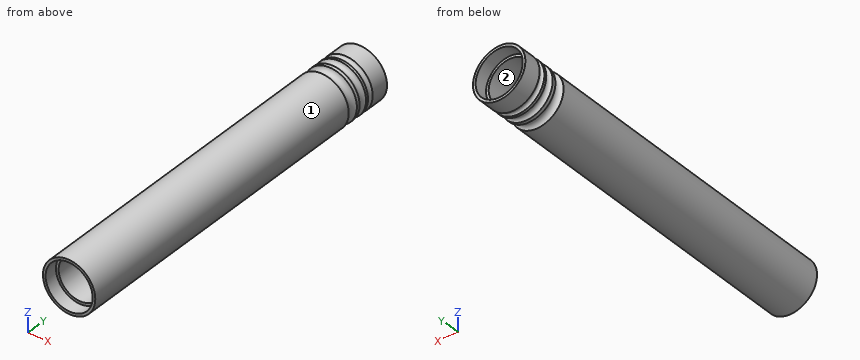
```python
from build123d import *

# Parameters (mm, degrees)
F0_R     = 25
F0_R_2   = 20
F1_DEPTH = 350
F2_R     = 22.5
F2_R_2   = 20
F3_DEPTH = 12.5
F4_R     = 22.5
F4_R_2   = 20
F5_DEPTH = 12.5
F6_R     = 3
F6_R_2   = 4
F6_R_3   = 5


with BuildPart() as f1:
    # F0 (on Front) → F1 (new body)
    with BuildSketch(Plane.XZ):
        Circle(F0_R)
        Circle(F0_R_2, mode=Mode.SUBTRACT)
    extrude(amount=F1_DEPTH)

    # F2 (on face) → F3 (cut)
    with BuildSketch(Plane.XZ.offset(350)):
        Circle(F2_R)
        Circle(F2_R_2, mode=Mode.SUBTRACT)
    extrude(amount=-F3_DEPTH, mode=Mode.SUBTRACT)

    # F4 (on face) → F5 (cut)
    with BuildSketch(Plane(origin=(0, 0, 0), x_dir=(-1, 0, 0), z_dir=(0, 1, 0))):
        Circle(F4_R)
        Circle(F4_R_2, mode=Mode.SUBTRACT)
    extrude(amount=-F5_DEPTH, mode=Mode.SUBTRACT)

    # F6 (on Right) → F7 (revolve, cut)
    with BuildSketch(Plane.YZ):
        with Locations((-20, 26)):
            Circle(F6_R)
        with Locations((-29, 26)):
            Circle(F6_R_2)
        with Locations((-41, 26)):
            Circle(F6_R_3)
    revolve(axis=Axis((0, 0, 0), (0, 1, 0)), mode=Mode.SUBTRACT)


solid = f1.part
```
Geometry check sheet. Reference: the model listing, model coordinates, mm. Face numbers are marked on the shaded views. Round coordinates to 2 decimals unless told otherwise and drop trailing zeros. Loops run counter-clockwise (first coordinate to the right, second up) from the corner with the lowest first, then second, coordinate; pieces in that order, holes last. Notation, with made-up numbers: (84, 57) - (111, 57) arc R22 cw to (111, 88) - close; hole circle Ø6 at (42, 55). An arc over 180 degrees is marked (long way). Use a Markdown table: item, result.
Q1. Cross-section at C-C on y = -153. Record the cut outline in (x, z), plus the area to 3 significant figures.
Solutions:
| item | result |
|---|---|
| outline | circle Ø50 at (0, 0); hole circle Ø40 at (0, 0) |
| area | 707 mm2 |
Q2. Cross-section at A-A on x = 0. Record the cut outline in (y, z).
Solutions:
| item | result |
|---|---|
| outline | (-350, -25) - (-45.9, -25) arc R5 cw to (-36.1, -25) - (-32.87, -25) arc R4 cw to (-25.13, -25) - (-22.83, -25) arc R3 cw to (-17.17, -25) - (0, -25) - (0, -22.5) - (-12.5, -22.5) - (-12.5, -20) - (-337.5, -20) - (-337.5, -22.5) - (-350, -22.5) - close; (-350, 22.5) - (-337.5, 22.5) - (-337.5, 20) - (-12.5, 20) - (-12.5, 22.5) - (0, 22.5) - (0, 25) - (-17.17, 25) arc R3 cw to (-22.83, 25) - (-25.13, 25) arc R4 cw to (-32.87, 25) - (-36.1, 25) arc R5 cw to (-45.9, 25) - (-350, 25) - close |
Q3. Material ranges on line 1 (Y direction, x = -19.5, z = -11); line 2 (Y direction, x = 12, z = 19.5); line 3 (Z direction, x = 0, y = -10), recorded low to high.
Solutions:
| item | result |
|---|---|
| line 1 | y = -337.5 to -44.46, -37.54 to -30.72, -27.28 to -12.5 |
| line 2 | y = -350 to -44.92, -37.08 to -31.52, -26.48 to 0 |
| line 3 | z = -25 to -22.5, 22.5 to 25 |
Q4. Draft check along X on the marked faces 1 and 2. Enter one of: released by +X, released by -X, zero draft, split by the parting line, or undercut.
Solutions:
| item | result |
|---|---|
| face 1 | split by the parting line |
| face 2 | undercut |
Q5. Cross-section at B-B on z = 0. Record the cut outline in (x, y).
Solutions:
| item | result |
|---|---|
| outline | (-25, -350) - (-22.5, -350) - (-22.5, -337.5) - (-20, -337.5) - (-20, -12.5) - (-22.5, -12.5) - (-22.5, 0) - (-25, 0) - (-25, -17.17) arc R3 cw to (-25, -22.83) - (-25, -25.13) arc R4 cw to (-25, -32.87) - (-25, -36.1) arc R5 cw to (-25, -45.9) - close; (20, -337.5) - (22.5, -337.5) - (22.5, -350) - (25, -350) - (25, -45.9) arc R5 cw to (25, -36.1) - (25, -32.87) arc R4 cw to (25, -25.13) - (25, -22.83) arc R3 cw to (25, -17.17) - (25, 0) - (22.5, 0) - (22.5, -12.5) - (20, -12.5) - close |
Q6. Go/stop test with flat-tipped pins: P1, Ø3, axis at x = -10.5, z = 14, coming from the +Y side; P2, Ø3, axis at y = -273, z = -3.5, coming from the +X side; P3, Ø8, axis at y = -299.5, z = 15, coming from the -X side; P4, Ø2, axis at x = -18, y = -195, coming from the +Z side. Record where each tip stops, or that it passes through.
Solutions:
| item | result |
|---|---|
| P1 | passes through |
| P2 | stops at x = 24.92 |
| P3 | stops at x = -22.45 |
| P4 | stops at z = 18.33 |
